```python
from build123d import *
from build123d.topology import SkipClean

# Parameters (mm, degrees)
SKETCH_1_R          = 7.6
EXTRUDE_1_DEPTH     = 5
SKETCH_2_W          = 18
SKETCH_2_H          = 5
EXTRUDE_2_DEPTH     = 15
EXTRUDE_3_DEPTH     = 3
SKETCH_5_W          = 3.5
SKETCH_5_H          = 5
EXTRUDE_4_DEPTH     = 12
SKETCH_3_R          = 4.1
CUT_EXTRUDE_1_DEPTH = 32.913946794
FILLET_4_R          = 1
SKETCH_6_W          = 25
SKETCH_6_H          = 12
SKETCH_6_R          = 4.1
EXTRUDE_5_DEPTH     = 4
FILLET_5_R          = 3
SKETCH_7_R          = 8.4
EXTRUDE_6_DEPTH     = 26.7
SKETCH_9_R          = 8.4
EXTRUDE_8_DEPTH     = 31.7
SKETCH_10_R         = 2.05
CUT_EXTRUDE_2_DEPTH = 5


with BuildPart() as part:
    # ｽｹｯﾁ1 → ﾎﾞｽ - 押し出し1 (new body)
    with BuildSketch(Plane(origin=(0, 0, 0), x_dir=(1, 0, 0), z_dir=(0, 1, 0))):
        with BuildLine():
            Line((-9, 0), (-9, -9))
            Line((-9, -9), (9, -9))
            Line((9, -9), (9, 0))
            ThreePointArc((9, 0), (0, 9), (-9, 0))
        make_face()
        with Locations(Location((0, 0, 0), (0, 0, 270))):
            Circle(SKETCH_1_R, mode=Mode.SUBTRACT)
    extrude(amount=EXTRUDE_1_DEPTH)

    # ｽｹｯﾁ2 → ﾎﾞｽ - 押し出し2 (add)
    with BuildSketch(Plane(origin=(0, 5, 0), x_dir=(1, 0, 0), z_dir=(0, 1, 0))):
        with Locations((0, -6.5)):
            Rectangle(SKETCH_2_W, SKETCH_2_H)
    extrude(amount=EXTRUDE_2_DEPTH)

    # ｽｹｯﾁ4 → ﾎﾞｽ - 押し出し3 (add)
    with BuildSketch(Plane(origin=(0, 5, 0), x_dir=(1, 0, 0), z_dir=(0, 1, 0))):
        with BuildLine():
            Line((-12.5, 0), (-12.5, -9))
            Line((-12.5, -9), (12.5, -9))
            Line((12.5, -9), (12.5, 0))
            ThreePointArc((12.5, 0), (0, 12.5), (-12.5, 0))
        make_face()
    extrude(amount=EXTRUDE_3_DEPTH)

    # ｽｹｯﾁ5 → ﾎﾞｽ - 押し出し4 (add)
    with BuildSketch(Plane(origin=(0, 8, 0), x_dir=(1, 0, 0), z_dir=(0, 1, 0))):
        with Locations((-10.75, -6.5)):
            Rectangle(SKETCH_5_W, SKETCH_5_H)
        with Locations((10.75, -6.5)):
            Rectangle(SKETCH_5_W, SKETCH_5_H)
    extrude(amount=EXTRUDE_4_DEPTH)

    # ｽｹｯﾁ3 → ｶｯﾄ - 押し出し1 (cut, through all)
    with BuildSketch(Plane.XY.offset(9)):
        with Locations((-6, 14)):
            Circle(SKETCH_3_R)
        with Locations((6, 14)):
            Circle(SKETCH_3_R)
    extrude(amount=-CUT_EXTRUDE_1_DEPTH, mode=Mode.SUBTRACT)

    # ﾌｨﾚｯﾄ4
    fillet_4_edges = [part.edges().sort_by_distance(p)[0] for p in [
        (9, 2.5, 9),
        (-9, 2.5, 9),
    ]]
    fillet(fillet_4_edges, radius=FILLET_4_R)

    # ｽｹｯﾁ6 → ﾎﾞｽ - 押し出し5 (add)
    with SkipClean():  # the faces are left unmerged after this step: merging them gives an invalid solid
        with BuildSketch(Plane(origin=(0, 0, 4), x_dir=(-1, 0, 0), z_dir=(0, 0, -1))):
            with Locations((0, 14)):
                Rectangle(SKETCH_6_W, SKETCH_6_H)
            with Locations((-6, 14)):
                Circle(SKETCH_6_R, mode=Mode.SUBTRACT)
            with Locations(Location((6, 14, 0), (0, 0, 180))):
                Circle(SKETCH_6_R, mode=Mode.SUBTRACT)
        extrude(amount=EXTRUDE_5_DEPTH)
    add(part.part.scale(1), mode=Mode.REPLACE)  # the faces are merged on a copy

    # ﾌｨﾚｯﾄ5
    fillet_5_edges = [part.edges().sort_by_distance(p)[0] for p in [
        (-12.5, 20, 4.5),
        (12.5, 20, 4.5),
    ]]
    fillet(fillet_5_edges, radius=FILLET_5_R)

    # ｽｹｯﾁ7 → ﾎﾞｽ - 押し出し6 (add)
    with SkipClean():  # the faces are left unmerged after this step: merging them gives an invalid solid
        with BuildSketch(Plane.XZ):
            with BuildLine():
                Line((8, 9), (-8, 9))
                ThreePointArc((-8, 9), (-8.707106781, 8.707106781), (-9, 8))
                Line((-9, 8), (-9, 0))
                ThreePointArc((-9, 0), (0, -9), (9, 0))
                Line((9, 0), (9, 8))
                ThreePointArc((9, 8), (8.707106781, 8.707106781), (8, 9))
            make_face()
            with Locations(Location((0, 0, 0), (0, 0, 270))):
                Circle(SKETCH_7_R, mode=Mode.SUBTRACT)
        extrude(amount=EXTRUDE_6_DEPTH)

    # ｽｹｯﾁ9 → ﾎﾞｽ - 押し出し8 (add)
    with SkipClean():  # the faces are left unmerged after this step: merging them gives an invalid solid
        with BuildSketch(Plane.XZ.offset(-5)):
            Circle(SKETCH_9_R)
        extrude(amount=EXTRUDE_8_DEPTH)

    # ｽｹｯﾁ10 → ｶｯﾄ - 押し出し2 (cut)
    with SkipClean():  # the faces are left unmerged after this step: merging them gives an invalid solid
        with BuildSketch(Plane.XZ.offset(26.7)):
            with Locations(Location((0, 0, 0), (0, 0, 270))):
                Circle(SKETCH_10_R)
        extrude(amount=-CUT_EXTRUDE_2_DEPTH, mode=Mode.SUBTRACT)


solid = part.part
```
Model file for the job. Use its own axes, mm. A direction names the side the tool comes from. Coordinates: 2 decimals unless noted, no trailing zeros. Order: outer loops, then holes, each group sorted by start corner. A loop starts at its lowest first (then second) coordinate and runs counter-clockwise, first axis right, second up. Notation, with made-up numbers: (66.5, 74) -> (85.5, 74) arc R24 cw to (85.5, 104) -> close; hole circle Ø1 at (50, 56). An arc over 180 degrees is marked (long way). Answer as a JSON object with one key per item and string values. Group by question number.
1) Cut at D-D, the plane x = 0. Write the cut outline in (y, z).
2) Cut at A-A, the plane y = 14. Write the cut outline in (x, z), then the cut area to 3 significant figures.
3) Which spindle directions (+Z, -Z, +X, -X, +Y, -Y) get a long thin tool onto all of the face, cutting with end or side? Do faces 5 (the face through (-8.699, -10.628, 8.715)), 6 (the face through (0, 14, 0)), 7 (the face through (9, -11, 4)). Say none if no direction does.
4) Flat gauge pins, fed straight in: pin 1 (12 mm diameter, centred on x = 8.5, y = -4, fed in from -Z); pin 2 (4 mm diameter, centred on x = -3, z = -4, fed in from +Y); pin 3 (1.5 mm diameter, centred on x = -1, y = -18, fed in from -Z). Where does each tip first touch, or does it go through?
5) Cut at B-B, the plane z = 4.5. Write the cut outline in (x, y).
6) Drill centre lines: L1, parallel to X at y = 14, z = 1.1; L2, parallel to Y at x = -6, z = 0.95; L3, parallel to Z at x = -6.25, y = 9. Where is each one in solid material? Low to high.
7) Cut at C-C, the plane x = 6. Write the cut outline in (y, z), then the cut area to 3 significant figures.
8) Pull direction Z, two halves, no side cores. Call faces 1 (the face through (8.715, -10.628, 8.699)), 2 (the face through (2.033, -24.235, 0.267)), 3 (the face through (12.5, 11, 5)), 4 (the face through (0, -21.7, 0)): +Z half, -Z half, draft (parallel to the pull), parting line (faces both ways), or undercut.
Check values:
{
 "1": {"outline": "(-26.7, -9) -> (5, -9) -> (5, -12.5) -> (8, -12.5) -> (8, 0) -> (20, 0) -> (20, 9) -> (-26.7, 9) -> (-26.7, 2.05) -> (-21.7, 2.05) -> (-21.7, -2.05) -> (-26.7, -2.05) -> close"},
 "2": {"outline": "(-12.5, 0) -> (-10.1, 0) -> (-10.1, 9) -> (-12.5, 9) -> close; (-1.9, 0) -> (1.9, 0) -> (1.9, 9) -> (-1.9, 9) -> close; (10.1, 0) -> (12.5, 0) -> (12.5, 9) -> (10.1, 9) -> close", "area": "77.4 mm²"},
 "3": {"face 5": "+Z, -X, -Y", "face 6": "-Z, +X, -X, +Y", "face 7": "+Z, -Z, +X, -Y"},
 "4": {"pin 1": "stops at z = -8.65", "pin 2": "stops at y = 8", "pin 3": "stops at z = -9"},
 "5": {"outline": "(-12.5, 5) -> (-9, 5) -> (-9, -26.7) -> (9, -26.7) -> (9, 5) -> (12.5, 5) -> (12.5, 17) arc R3 ccw to (9.5, 20) -> (-9.5, 20) arc R3 ccw to (-12.5, 17) -> close; hole circle Ø8.2 at (-6, 14); hole circle Ø8.2 at (6, 14)"},
 "6": {"L1": "x = -12.5 to -10.1, -1.9 to 1.9, 10.1 to 12.5", "L2": "y = -26.7 to 9.9, 18.1 to 20", "L3": "z = 0 to 9"},
 "7": {"outline": "(-26.7, -6.71) -> (5, -6.71) -> (5, -10.97) -> (8, -10.97) -> (8, 0) -> (9.9, 0) -> (9.9, 9) -> (-26.7, 9) -> close; (18.1, 0) -> (20, 0) -> (20, 9) -> (18.1, 9) -> close", "area": "592 mm²"},
 "8": {"face 1": "+Z half", "face 2": "undercut", "face 3": "draft", "face 4": "undercut"}
}
